from build123d import *

# Parameters (mm, degrees)
SKETCH1_R           = 2.05
SKETCH1_W           = 6
SKETCH1_H           = 3
BOSS_EXTRUDE1_DEPTH = 3
FILLET1_R           = 5


with BuildPart() as part:
    # Sketch1 → Boss-Extrude1 (new body)
    with BuildSketch(Plane.XY):
        Polygon((-43.603832711, -10.844440202), (-76, -10.844440202), (-76, 59.155559798), (-46, 102), (-46, 167), (0, 167), (0, 121.42828657), (-43.603832711, 59.155559798), (-43.603832711, 39.727273228), align=None)
        with Locations((-71, 34.155559798)):
            Circle(SKETCH1_R, mode=Mode.SUBTRACT)
        with Locations((-71, -5.844440202)):
            Circle(SKETCH1_R, mode=Mode.SUBTRACT)
        with Locations((-38, 157)):
            Rectangle(SKETCH1_W, SKETCH1_H, mode=Mode.SUBTRACT)
        with Locations((-8, 157)):
            Rectangle(SKETCH1_W, SKETCH1_H, mode=Mode.SUBTRACT)
    extrude(amount=BOSS_EXTRUDE1_DEPTH)

    # Fillet1
    fillet1_edges = [part.edges().sort_by_distance(p)[0] for p in [
        (-43.603832711, 59.155559798, 1.5),
        (-43.603832711, -10.844440202, 1.5),
        (-76, -10.844440202, 1.5),
        (-76, 59.155559798, 1.5),
        (-46, 102, 1.5),
        (-46, 167, 1.5),
        (0, 167, 1.5),
        (0, 121.42828657, 1.5),
    ]]
    fillet(fillet1_edges, radius=FILLET1_R)


solid = part.part
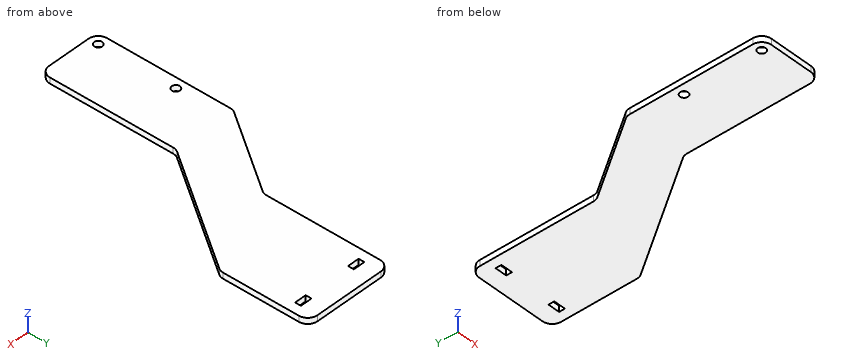
Read the model definition and answer for the solid it produces. Units are mm, in the model's axes. Coordinates: 2 decimals unless noted, no trailing zeros. Loops run counter-clockwise (first coordinate to the right, second up) from the corner with the lowest first, then second, coordinate; pieces in that order, holes last.
Q1. Consider probe 1 along Y at (x, z) = (-71, 0.7); probe 2 along X at (y, z) = (127, 0.45); probe 3 along X at (y, z) = (49, 0.5). Determine where each line is inside the solid, lowest interval first.
Q2. Each of these flat-tipped pins is pushed along its axis until it touches: pin 1 Ø0.9 at (y, z) = (12, 1) entering from +X; pin 2 Ø1.5 at (y, z) = (140.5, 1) entering from -X; pin 3 Ø4 at (x, y) = (-58, 37.5) entering from -Z; pin 4 Ø3.5 at (x, y) = (-71, 34.16) entering from -Z. Where does it stop, or does it pass through?
Q3. The part is cut by section A-A on z = 1.15. Write down the section's boundary in (x, y), and give its area (3 significant figures).
Q4. The part is cut by section B-B on y = 15.5. Write down the section's boundary in (x, z), and give its area (3 significant figures).
Results below:
1. probe 1: y = -10.84 to -7.89, -3.79 to 32.11, 36.21 to 66.3
1. probe 2: x = -46 to 0
1. probe 3: x = -76 to -43.6
2. pin 1: stops at x = -43.6
2. pin 2: stops at x = -46
2. pin 3: stops at z = 0
2. pin 4: passes through
3. outline: (-76, -5.84) arc R5 ccw to (-71, -10.84) - (-48.6, -10.84) arc R5 ccw to (-43.6, -5.84) - (-43.6, 57.58) arc R5 cw to (-42.7, 60.45) - (-0.9, 120.14) arc R5 ccw to (0, 123) - (0, 162) arc R5 ccw to (-5, 167) - (-41, 167) arc R5 ccw to (-46, 162) - (-46, 103.58) arc R5 cw to (-46.9, 100.71) - (-75.1, 60.45) arc R5 ccw to (-76, 57.58) - close; hole circle Ø4.1 at (-71, -5.84); hole circle Ø4.1 at (-71, 34.16); hole (-41, 155.5) - (-35, 155.5) - (-35, 158.5) - (-41, 158.5) - close; hole (-11, 155.5) - (-5, 155.5) - (-5, 158.5) - (-11, 158.5) - close
3. area: 6,430 mm2
4. outline: (-76, 0) - (-43.6, 0) - (-43.6, 3) - (-76, 3) - close
4. area: 97.2 mm2
